Autodesk Inventor part; units mm, degrees
ref_plane "YZ Plane" through (0, 0, 0) normal (1, 0, 0) x (0, 1, 0)
ref_plane "XZ Plane" through (0, 0, 0) normal (0, 1, 0) x (-1, 0, 0)
ref_plane "XY Plane" through (0, 0, 0) normal (0, 0, 1) x (1, 0, 0)
sketch "Sketch1" plane through (0, 0, 0) normal (0, 0, 1) x (1, 0, 0)
  circle A0 centre (0, 0) radius 60
  dimension "d0" = 120
extrude "Extrusion1" add sketch "Sketch1" along normal blind 10
sketch "Sketch2" plane through (0, 0, 10) normal (0, 0, 1) x (1, 0, 0)
  circle A0 centre (0, 0) radius 31.5
  dimension "d3" = 63
extrude "Extrusion2" add sketch "Sketch2" along normal blind 17.4
sketch "Sketch3" plane through (0, 0, 27.4) normal (0, 0, 1) x (1, 0, 0)
  circle A0 centre (-14.5, 14.5) radius 2
  circle A1 centre (14.5, 14.5) radius 2
  circle A2 centre (14.5, -14.5) radius 2
  circle A3 centre (-14.5, -14.5) radius 2
  point P0 (0, 0)
  dimension "d6" = 4
  dimension "d7" = 4
  dimension "d8" = 4
  dimension "d9" = 4
  dimension "d10" = 29
  dimension "d11" = 29
  dimension "d12" = 29
  dimension "d13" = 29
  dimension "d18" = 20.5061
  dimension "d19" = 20.5061
  dimension "d20" = 20.5061
extrude "Extrusion3" cut sketch "Sketch3" against normal through all
sketch "Sketch4" plane through (0, 0, 0) normal (0, 0, -1) x (-1, 0, 0)
  circle A0 centre (0, 0) radius 44
  dimension "d23" = 88
extrude "Extrusion4" add sketch "Sketch4" along normal blind 2
sketch "Sketch5" plane through (0, 0, -2) normal (0, 0, -1) x (-1, 0, 0)
  circle A0 centre (0, 0) radius 26
  dimension "d26" = 52
extrude "Extrusion5" cut sketch "Sketch5" against normal blind 24
sketch "Sketch6" plane through (0, 0, 0) normal (0, 0, -1) x (-1, 0, 0)
  circle A0 centre (-45.068, -26.02) radius 4.2
  circle A1 centre (45.068, -26.02) radius 4.2
  circle A2 centre (0, 52) radius 4.2
  circle A3 centre (0, 0) radius 44
  dimension "d29" = 8.4
  dimension "d30" = 8.4
  dimension "d31" = 8.4
extrude "Extrusion6" cut sketch "Sketch6" against normal blind 10 contours A0 | A1 | A2
properties part number "tampa traseira acoplada final"
Can you work these out from the model? Positions are in its coordinate system, mm. A direction names the side the tool comes from. Give positions to 0.01 mm unless a question says otherwise; leave off trailing zeros. Loops run counter-clockwise (first coordinate to the right, second up) from the corner with the lowest first, then second, coordinate; pieces in that order, holes last. Notation, with made-up numbers: (-31, -27) -> (-16, -27) arc R10 ccw to (-16, -22) -> close; hole circle Ø9 at (33.25, 25.5). An arc over 180 degrees is marked (long way). Use one line per item in the form item = value.
1) If we section it at A-A (y = 14.5): Please give me the cut outline in (x, z), plus the area to 3 significant figures.
Answers:
outline = (-58.22, 0) -> (-41.54, 0) -> (-41.54, -2) -> (-21.58, -2) -> (-21.58, 22) -> (-16.5, 22) -> (-16.5, 27.4) -> (-27.96, 27.4) -> (-27.96, 10) -> (-58.22, 10) -> close; (-12.5, 22) -> (12.5, 22) -> (12.5, 27.4) -> (-12.5, 27.4) -> close; (16.5, 22) -> (21.58, 22) -> (21.58, -2) -> (41.54, -2) -> (41.54, 0) -> (58.22, 0) -> (58.22, 10) -> (27.96, 10) -> (27.96, 27.4) -> (16.5, 27.4) -> close
area = 1,220 mm²
2) For faces 5 (the face through (-19, -19, -2)), 6 (the face through (9.538, 42.954, -0.986)), 7 (the face through (26, -26, 10)), which set-ups out of +Z, -Z, +X, -X, +Y, -Y let a thin tool reach every point of the face, with its end or its side?
Answers:
face_5 = -Z, +X, -X, +Y, -Y
face_6 = -Z
face_7 = +Z
3) We'd pull the mould along X, two halves only. Please class faces 1 (the face through (20.633, -15.821, 9.832)), 2 (the face through (-40.3, 18.1, 0)), 3 (the face through (41.06, -24.76, 4.93)), 4 (the face through (-4.101, -31.232, 18.578)): released by +X, released by -X, zero draft, split by the parting line, or undercut.
Answers:
face_1 = undercut
face_2 = zero draft
face_3 = undercut
face_4 = split by the parting line
4) If we section it at B-B (z = 24.25): Please give me the cut outline in (x, y), plus the area to 3 significant figures.
Answers:
outline = circle Ø63 at (0, 0); hole circle Ø4 at (-14.5, -14.5); hole circle Ø4 at (-14.5, 14.5); hole circle Ø4 at (14.5, -14.5); hole circle Ø4 at (14.5, 14.5)
area = 3,070 mm²
5) I need wall thicknesses on line 1 along Y through (x, z) = (0, 5.5); line 2 along Z through (x, y) = (19, 55.5); line 3 along Z through (x, y) = (-3, -11). Which ranges of each line are inside material? Lowest first, please.
Answers:
line_1 = -60 to -26, 26 to 47.8, 56.2 to 60
line_2 = 0 to 10
line_3 = 22 to 27.4
6) If we section it at C-C (y = 52): Please give me the cut outline in (x, z).
Answers:
outline = (-29.93, 0) -> (-4.2, 0) -> (-4.2, 10) -> (-29.93, 10) -> close; (4.2, 0) -> (29.93, 0) -> (29.93, 10) -> (4.2, 10) -> close
7) Will these pins go through, and if not, where does the flat tip stop? pin 1 (5 mm diameter, centred on x = -2.5, z = 20, fed in from -Y); pin 2 (5 mm diameter, centred on x = 35.5, y = 32.5, fed in from -Z); pin 3 (3 mm diameter, centred on x = 48, z = 11, fed in from +Y).
Answers:
pin_1 = -31.5
pin_2 = 0
pin_3 = 37.44
